Input: part model. Units: mm. Frame: model coordinates. Face numbers are marked on the shaded views. A direction names the side the tool comes from. Round coordinates to 2 decimals unless told otherwise and drop trailing zeros. Write each loop counter-clockwise with the first axis right and the second up, starting at its lowest first coordinate (ties: lowest second). Pieces come first, ordered by that corner, then holes. Notation, with made-up numbers: (69.5, 51.25) -> (76.5, 51.25) arc R15 cw to (76.5, 77.25) -> close; hole circle Ø9 at (75, -4.5). An arc over 180 degrees is marked (long way). Write item = value, one per line.
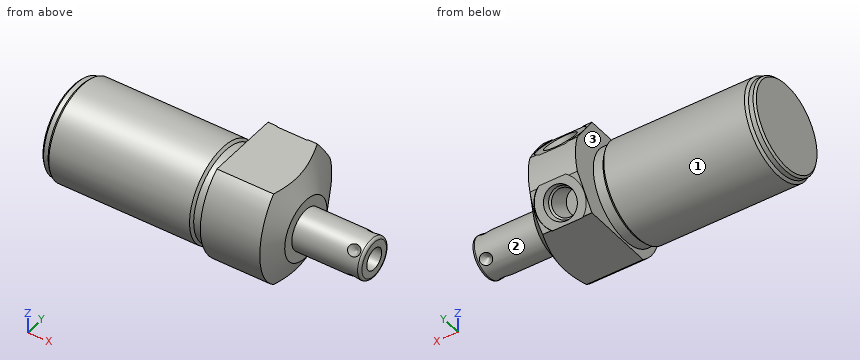
```python
from build123d import *

# Parameters (mm, degrees)
SKETCH1_R           = 23.8125
EXTRUDE1_DEPTH      = 27.7876
EXTRUDE1_DEPTH_BACK = 63.5
CUT_EXTRUDE1_REACH  = 65.5
SKETCH2_R           = 23.8125
SKETCH2_R_2         = 18.8595
CUT_EXTRUDE3_START  = -27.7876
SKETCH4_R           = 28.575
CUT_EXTRUDE3_DEPTH  = 27.7876
SKETCH18_R          = 9.525
CUT_EXTRUDE4_DEPTH  = 0.254
SKETCH19_R          = 9.525
CUT_EXTRUDE5_DEPTH  = 0.254
CHAMFER1_SIZE       = 0.762
CIRPATTERN1_COUNT   = 4


with BuildPart() as part:
    # Sketch1 → Extrude1 (new body, two sides)
    with BuildSketch(Plane(origin=(0, 0, 0), x_dir=(0, 0, -1), z_dir=(1, 0, 0))) as extrude1_sk:
        Circle(SKETCH1_R)
    extrude(amount=EXTRUDE1_DEPTH)
    extrude(extrude1_sk.sketch, amount=-EXTRUDE1_DEPTH_BACK)

    # Sketch2 → Cut-Extrude1 (cut, up to next)
    with BuildSketch(Plane(origin=(0, 0, 0), x_dir=(0, 0, -1), z_dir=(1, 0, 0)), mode=Mode.PRIVATE) as cut_extrude1_sk1:
        Circle(SKETCH2_R)
        with Locations((0, -4.191)):
            Circle(SKETCH2_R_2, mode=Mode.SUBTRACT)
    cut_extrude1_tool1 = extrude(cut_extrude1_sk1.sketch, amount=-CUT_EXTRUDE1_REACH, mode=Mode.PRIVATE) & part.part
    add(cut_extrude1_tool1.solids().sort_by_distance((0, 0, 23.138981))[0], mode=Mode.SUBTRACT)

    # Sketch4 → Cut-Extrude3 (cut)
    with BuildSketch(Plane.ZY.offset(CUT_EXTRUDE3_START)):
        Circle(SKETCH4_R)
        with BuildLine():
            Line((18.923, -14.455283714), (18.923, 14.465869871))
            Line((18.923, 14.465869871), (0, 27.715897117))
            Line((0, 27.715897117), (-18.923, 14.465869871))
            Line((-18.923, 14.465869871), (-18.923, -14.455283714))
            ThreePointArc((-18.923, -14.455283714), (0, -23.8125), (18.923, -14.455283714))
        make_face(mode=Mode.SUBTRACT)
    extrude(amount=CUT_EXTRUDE3_DEPTH, mode=Mode.SUBTRACT)

    # Sketch6 → Cut-Revolve2 (revolve, cut)
    with BuildSketch(Plane.XY, mode=Mode.PRIVATE) as cut_revolve2_sk:
        Polygon((4.764025965, 47.625), (27.7876, 7.747), (27.7876, 47.625), align=None)
    revolve(cut_revolve2_sk.sketch.rotate(Axis((3.612847264, -4.191, 0), (1, 0, 0)), 270), axis=Axis((3.612847264, -4.191, 0), (1, 0, 0)), mode=Mode.SUBTRACT)  # turned: the seam where the file's is

    # S2D0002 → Cut-Revolve3 (revolve, cut)
    with BuildSketch(Plane(origin=(9.652, 18.394824642, 12.869035589), x_dir=(0, 0.573576436, -0.819152044), z_dir=(1, 0, 0))):
        Polygon((0, 0), (6.1849, 0), (5.642306865, -2.5527), (4.9784, -3.216606865), (4.9784, -13.462), (0, -13.462), align=None)
    revolve(axis=Axis((9.652, 6.816028581, 4.761475303), (0, 0.819152044, 0.573576436)), mode=Mode.SUBTRACT)

    # Sketch8 → Cut-Revolve4 (revolve, cut)
    with BuildSketch(Plane(origin=(9.652, 18.394824642, -12.869035589), x_dir=(0, -0.573576436, -0.819152044), z_dir=(1, 0, 0))):
        Polygon((0, 0), (6.1849, 0), (5.642306865, -2.5527), (4.9784, -3.216606865), (4.9784, -13.462), (0, -13.462), align=None)
    revolve(axis=Axis((9.652, 6.816028581, -4.761475303), (0, 0.819152044, -0.573576436)), mode=Mode.SUBTRACT)

    # Sketch18 → Cut-Extrude4 (cut)
    with BuildSketch(Plane(origin=(0, 18.59764611, 13.022211999), x_dir=(1, 0, 0), z_dir=(0, 0.819152044, 0.573576436))):
        with Locations((9.652, 0.009141155)):
            Circle(SKETCH18_R)
    extrude(amount=-CUT_EXTRUDE4_DEPTH, mode=Mode.SUBTRACT)

    # Sketch19 → Cut-Extrude5 (cut)
    with BuildSketch(Plane(origin=(0, 18.59764611, -13.022211999), x_dir=(1, 0, 0), z_dir=(0, 0.819152044, -0.573576436))):
        with Locations((9.652, -0.009141155)):
            Circle(SKETCH19_R)
    extrude(amount=-CUT_EXTRUDE5_DEPTH, mode=Mode.SUBTRACT)

    # Sketch10 → Cut-Revolve6 (revolve, cut)
    with BuildSketch(Plane.XY, mode=Mode.PRIVATE) as cut_revolve6_sk:
        Polygon((0, 14.6685), (0, 13.716), (-3.81, 13.716), (-4.7625, 14.6685), align=None)
    revolve(cut_revolve6_sk.sketch.rotate(Axis((-5.000625, -4.191, 0), (1, 0, 0)), 90), axis=Axis((-5.000625, -4.191, 0), (1, 0, 0)), mode=Mode.SUBTRACT)  # turned: the seam where the file's is

    # Sketch12 → Cut-Revolve8 (revolve, cut)
    with BuildSketch(Plane.XY, mode=Mode.PRIVATE) as cut_revolve8_sk:
        Polygon((-63.5, 14.6685), (-63.5, 13.716), (-60.96, 13.716), (-60.0075, 14.6685), align=None)
    revolve(cut_revolve8_sk.sketch.rotate(Axis((-63.674625, -4.191, 0), (1, 0, 0)), 90), axis=Axis((-63.674625, -4.191, 0), (1, 0, 0)), mode=Mode.SUBTRACT)  # turned: the seam where the file's is

    # Chamfer1
    chamfer1_edges = [part.edges().sort_by_distance(p)[0] for p in [
        (-63.5, -4.191, -17.907),
    ]]
    chamfer(chamfer1_edges, length=CHAMFER1_SIZE)

    # Sketch13 → Revolve1 (revolve)
    with BuildSketch(Plane(origin=(0, 0, 0), x_dir=(0, -1, 0), z_dir=(0, 0, 1)), mode=Mode.PRIVATE) as revolve1_sk:
        with BuildLine():
            Line((4.191, 27.7876), (4.191, 54.6354))
            Line((4.191, 54.6354), (11.1125, 54.6354))
            ThreePointArc((11.1125, 54.6354), (11.83092049, 54.33782049), (12.1285, 53.6194))
            Line((12.1285, 53.6194), (12.1285, 27.7876))
            Line((12.1285, 27.7876), (4.191, 27.7876))
        make_face()
    revolve(revolve1_sk.sketch.rotate(Axis((26.44521, -4.191, 0), (1, 0, 0)), 270), axis=Axis((26.44521, -4.191, 0), (1, 0, 0)))  # turned: the seam where the file's is

    # S2D0001 → Cut-Revolve9 (revolve, cut)
    with BuildSketch(Plane(origin=(54.6354, -8.4074, 0), x_dir=(0, -1, 0), z_dir=(0, 0, 1)), mode=Mode.PRIVATE) as cut_revolve9_sk:
        Polygon((0, 0), (0, -15.24), (-4.2164, -17.773468714), (-4.2164, 0), align=None)
    revolve(cut_revolve9_sk.sketch.rotate(Axis((35.97325785, -4.191, 0), (1, 0, 0)), 270), axis=Axis((35.97325785, -4.191, 0), (1, 0, 0)), mode=Mode.SUBTRACT)  # turned: the seam where the file's is

    # Sketch16 → Cut-Revolve10 (revolve, cut)
    with BuildSketch(Plane(origin=(50.673, 1.421660076, -5.612660076), x_dir=(-1, 0, 0), z_dir=(0, -0.707106781, -0.707106781)), mode=Mode.PRIVATE) as cut_revolve10_sk:
        Polygon((0, 0), (2.413, 0), (0, -2.413), align=None)
    cut_revolve10 = revolve(cut_revolve10_sk.sketch.rotate(Axis((50.673, -2.1640922, -2.0269078), (0, 0.707106781, -0.707106781)), 90), axis=Axis((50.673, -2.1640922, -2.0269078), (0, 0.707106781, -0.707106781)), mode=Mode.SUBTRACT)  # turned: the seam where the file's is

    # CirPattern1: Cut-Revolve10 ×4 about axis
    cirpattern1_axis = Axis((26.44521, -4.191, 0), (-1, 0, 0))
    for i in range(1, CIRPATTERN1_COUNT):
        add(cut_revolve10.rotate(cirpattern1_axis, i * 360 / CIRPATTERN1_COUNT), mode=Mode.SUBTRACT)


solid = part.part
```
1) Line query: L1, parallel to Y at x = 50.5, z = 0; L2, parallel to Y at x = 41, z = 1; L3, parallel to X at y = 15, z = 13.5. Output: solid intervals per line, ascending. Write a range as from..to.
Solutions:
L1 = -12.13..-8.41, 0.03..3.75
L2 = -12.07..-8.29, -0.09..3.68
L3 = 0..4.54, 14.76..21.13
2) Access query for the marked faces 1, 2 and 3. Directions: +Z, -Z, +X, -X, +Y, -Y. A direction counts if a zero-diameter tool reaches every point of the face in a straight line with its end or side. Return the directions, or none.
Solutions:
face_1 = -X
face_2 = +X
face_3 = none
3) Cut plane A-A (x = -22). Return the cut outline in (y, z).
Solutions:
outline = circle Ø37.72 at (-4.19, 0)
4) First-contact query: P1, Ø1, axis at x = -5, z = 13.5, coming from the -Y side; P2, Ø2, axis at x = 17.5, z = 0.5, coming from the +Y side; P3, Ø4, axis at y = 18.5, z = 12, coming from the -X side; P4, Ø7, axis at y = -2.5, z = 1, coming from the +X side. Flat tips, straight axial feed; report the tip coordinate or a pass-through.
Solutions:
P1 = -17.85
P2 = 23.81
P3 = 0
P4 = 54.64
